Verification items for the finished model (mm, model axes). A direction names the side the tool comes from. Give positions to 0.01 mm unless a question says otherwise; leave off trailing zeros. Order: outer loops, then holes, each group sorted by start corner. A loop starts at its lowest first (then second) coordinate and runs counter-clockwise, first axis right, second up. Notation, with made-up numbers: M -16,76.25 L 12,76.25 A21 ccw 12,98.25 Z; hole C 49,-11.5 d8. An arc over 180 degrees is marked long. Answer as a JSON object with one key per item and string values.
```python
from build123d import *

# Parameters (mm, degrees)
SKETCH1_R             = 1.75
BOSS_EXTRUDE1_DEPTH   = 11
BOSS_EXTRUDE1_2_DEPTH = 11
BOSS_EXTRUDE2_START   = 11
SKETCH1_3_W           = 50
SKETCH1_3_H           = 18
SKETCH1_3_R           = 1.75
BOSS_EXTRUDE2_DEPTH   = 6
SKETCH3_R             = 4.25
CUT_EXTRUDE1_DEPTH    = 5
SKETCH4_R             = 1.6
CUT_EXTRUDE2_DEPTH    = 42.548164821
CUT_EXTRUDE3_DEPTH    = 1.5


with BuildPart() as part:
    # Sketch1 → Boss-Extrude1 (new body)
    with BuildSketch(Plane.XY):
        with BuildLine():
            Line((18, 12.5), (-18, 12.5))
            ThreePointArc((-18, 12.5), (-21.5, 16), (-25, 12.5))
            Line((-25, 12.5), (-25, 9))
            Line((-25, 9), (25, 9))
            Line((25, 9), (25, 12.5))
            ThreePointArc((25, 12.5), (21.5, 16), (18, 12.5))
        make_face()
        with Locations((-21.5, 12.5)):
            Circle(SKETCH1_R, mode=Mode.SUBTRACT)
        with Locations((21.5, 12.5)):
            Circle(SKETCH1_R, mode=Mode.SUBTRACT)
    extrude(amount=BOSS_EXTRUDE1_DEPTH)



with BuildPart() as body_2:
    # Sketch1 → Boss-Extrude1 2 (new body)
    with BuildSketch(Plane.XY):
        with BuildLine():
            Line((25, -9), (-25, -9))
            Line((-25, -9), (-25, -12.5))
            ThreePointArc((-25, -12.5), (-21.5, -16), (-18, -12.5))
            Line((-18, -12.5), (18, -12.5))
            ThreePointArc((18, -12.5), (21.5, -16), (25, -12.5))
            Line((25, -12.5), (25, -9))
        make_face()
        with Locations((-21.5, -12.5)):
            Circle(SKETCH1_R, mode=Mode.SUBTRACT)
        with Locations((21.5, -12.5)):
            Circle(SKETCH1_R, mode=Mode.SUBTRACT)
    extrude(amount=BOSS_EXTRUDE1_2_DEPTH)


with BuildPart() as part_1:
    add(part.part)

    add(body_2.part)  # Boss-Extrude2 merges body 2
    # Sketch1<3> → Boss-Extrude2 (add)
    # profile 1 of 3: a face of its own
    with BuildSketch(Plane.XY.offset(BOSS_EXTRUDE2_START)):
        Rectangle(SKETCH1_3_W, SKETCH1_3_H)
    # profile 2 of 3: a face of its own
    with BuildSketch(Plane.XY.offset(BOSS_EXTRUDE2_START)):
        with BuildLine():
            Line((18, 12.5), (-18, 12.5))
            ThreePointArc((-18, 12.5), (-21.5, 16), (-25, 12.5))
            Line((-25, 12.5), (-25, 9))
            Line((-25, 9), (25, 9))
            Line((25, 9), (25, 12.5))
            ThreePointArc((25, 12.5), (21.5, 16), (18, 12.5))
        make_face()
        with Locations((-21.5, 12.5)):
            Circle(SKETCH1_3_R, mode=Mode.SUBTRACT)
        with Locations((21.5, 12.5)):
            Circle(SKETCH1_3_R, mode=Mode.SUBTRACT)
    # profile 3 of 3: a face of its own
    with BuildSketch(Plane.XY.offset(BOSS_EXTRUDE2_START)):
        with BuildLine():
            Line((25, -9), (-25, -9))
            Line((-25, -9), (-25, -12.5))
            ThreePointArc((-25, -12.5), (-21.5, -16), (-18, -12.5))
            Line((-18, -12.5), (18, -12.5))
            ThreePointArc((18, -12.5), (21.5, -16), (25, -12.5))
            Line((25, -12.5), (25, -9))
        make_face()
        with Locations((-21.5, -12.5)):
            Circle(SKETCH1_3_R, mode=Mode.SUBTRACT)
        with Locations((21.5, -12.5)):
            Circle(SKETCH1_3_R, mode=Mode.SUBTRACT)
    extrude(amount=BOSS_EXTRUDE2_DEPTH)

    # Sketch3 → Cut-Extrude1 (cut)
    with BuildSketch(Plane(origin=(0, 0, 11), x_dir=(-1, 0, 0), z_dir=(0, 0, -1))):
        with Locations((-15, 0)):
            Circle(SKETCH3_R)
    extrude(amount=-CUT_EXTRUDE1_DEPTH, mode=Mode.SUBTRACT)

    # Sketch4 → Cut-Extrude2 (cut, through all)
    with BuildSketch(Plane.XZ.offset(12.5)):
        with Locations(Location((-13, 7.5, 0), (0, 0, 270))):
            Circle(SKETCH4_R)
    extrude(amount=-CUT_EXTRUDE2_DEPTH, mode=Mode.SUBTRACT)

    # Sketch5 → Cut-Extrude3 (cut)
    with BuildSketch(Plane(origin=(0, 12.5, 0), x_dir=(1, 0, 0), z_dir=(0, 1, 0))):
        Polygon((-9.868012442, -9.567362395), (-9.643617868, -5.821300408), (-12.775605426, -3.753938013), (-16.131987558, -5.432637605), (-16.356382132, -9.178699592), (-13.224394574, -11.246061987), align=None)
    extrude(amount=-CUT_EXTRUDE3_DEPTH, mode=Mode.SUBTRACT)


solid = part_1.part
```
Q1. Section check B-B on z = 8. Record the cut outline in (x, y).
Resolved:
{"outline": "M -25,-12.5 A3.5 ccw -18,-12.5 L -14.52,-12.5 L -14.52,-9 L -25,-9 Z; M -25,9 L -14.52,9 L -14.52,11 L -16.29,11 L -16.29,12.5 L -18,12.5 A3.5 ccw -25,12.5 Z; M -11.48,-12.5 L 18,-12.5 A3.5 ccw 25,-12.5 L 25,-9 L -11.48,-9 Z; M -11.48,9 L 25,9 L 25,12.5 A3.5 ccw 18,12.5 L -9.77,12.5 L -9.77,11 L -11.48,11 Z; hole C -21.5,-12.5 d3.5; hole C -21.5,12.5 d3.5; hole C 21.5,-12.5 d3.5; hole C 21.5,12.5 d3.5"}
Q2. Section check D-D on z = 11.75. Record the cut outline in (x, y), then the cut area to 3 significant figures.
Resolved:
{"outline": "M -25,-12.5 A3.5 ccw -18,-12.5 L 18,-12.5 A3.5 ccw 25,-12.5 L 25,12.5 A3.5 ccw 18,12.5 L -18,12.5 A3.5 ccw -25,12.5 Z; hole C -21.5,-12.5 d3.5; hole C -21.5,12.5 d3.5; hole C 15,0 d8.5; hole C 21.5,-12.5 d3.5; hole C 21.5,12.5 d3.5", "area": "1,230 mm²"}
Q3. Material ranges on L1, parallel to Y at x = 21.5, z = 10.5; L2, parallel to X at y = 13.5, z = 2; L3, parallel to Y at x = -3.5, z = 3.25, recorded low to high.
Resolved:
{"L1": "y = -16 to -14.25, -10.75 to -9, 9 to 10.75, 14.25 to 16", "L2": "x = -24.85 to -22.94, -20.06 to -18.15, 18.15 to 20.06, 22.94 to 24.85", "L3": "y = -12.5 to -9, 9 to 12.5"}
Q4. Section check C-C on y = 0. Record the cut outline in (x, z).
Resolved:
{"outline": "M -25,11 L 10.75,11 L 10.75,16 L 19.25,16 L 19.25,11 L 25,11 L 25,17 L -25,17 Z"}
Q5. Gauge pin test, flat ends, axial feed: pin 1 Ø5.5 at (x, y) = (0, 3.5) entering from -Z; pin 2 Ø2.5 at (x, y) = (16, -2) entering from -Z; pin 3 Ø9 at (x, z) = (-1.5, 6) entering from +Y. Record the tip position at first contact, or that the pin passes through.
Resolved:
{"pin 1": "stops at z = 11", "pin 2": "stops at z = 16", "pin 3": "stops at y = 12.5"}
Q6. Release check for a two-part mould opening along Z. For faces 6 (the face through (0, 0, 17)), 7 (the face through (21.6, 16, 8.4)), 8 (the face through (15, 0, 16)), 9 (the face through (-11.19, 11.76, 4.8)) record: +Z half, -Z half, draft (parallel to the pull), parting line (faces both ways), or undercut.
Resolved:
{"face 6": "+Z half", "face 7": "draft", "face 8": "-Z half", "face 9": "undercut"}
Q7. Section check A-A on x = -21.5. Record the cut outline in (y, z).
Resolved:
{"outline": "M -16,0 L -14.25,0 L -14.25,17 L -16,17 Z; M -10.75,0 L -9,0 L -9,11 L 9,11 L 9,0 L 10.75,0 L 10.75,17 L -10.75,17 Z; M 14.25,0 L 16,0 L 16,17 L 14.25,17 Z"}
Q8. Tool access check on faces 1 (the face through (0, -12.5, 8)), 2 (the face through (0, -11, 0)), 3 (the face through (-23.25, 12.58, 8.38)), 4 (the face through (0, 0, 11)), 5 (the face through (-14.43, 11.76, 4.58)). Record the directions out of +Z, -Z, +X, -X, +Y, -Y that give a thin tool (end or side, any length) a straight path to the whole face; none if there is none.
Resolved:
{"face 1": "+Z, -Z, -Y", "face 2": "-Z, +X, -X, +Y, -Y", "face 3": "+Z, -Z", "face 4": "-Z, +X, -X", "face 5": "+Y"}
